from build123d import *

# Parameters (mm, degrees)
SHELL1_T  = -0.1
SKETCH4_W = 5
SKETCH4_H = 6


with BuildPart() as part:
    # Sketch3 → Revolve1 (revolve)
    with BuildSketch(Plane.XY):
        with BuildLine():
            Line((0, 0), (5, 0))
            ThreePointArc((5, 0), (3.535533906, 3.535533906), (0, 5))
            Line((0, 5), (0, 0))
        make_face()
    revolve(axis=Axis((0, 0, 0), (0, 1, 0)))

    # Shell1
    shell1_openings = [part.faces().sort_by_distance(p)[0] for p in [
        (0, 0, 0),
    ]]
    offset(amount=SHELL1_T, openings=shell1_openings, kind=Kind.INTERSECTION)

    # Sketch4 → Revolve2 (revolve)
    with BuildSketch(Plane.XY):
        with Locations((2.5, -3)):
            Rectangle(SKETCH4_W, SKETCH4_H)
    revolve(axis=Axis((0, -6, 0), (0, 1, 0)))


solid = part.part
Design review of the part built by this model. Coordinates are the model's own, in mm. Round coordinates to 2 decimals unless told otherwise and drop trailing zeros. Write each loop counter-clockwise with the first axis right and the second up, starting at its lowest first coordinate (ties: lowest second). Pieces come first, ordered by that corner, then holes. Notation, with made-up numbers: (-33, 8) - (-27, 8) arc R21 ccw to (-27, 33) - close; hole circle Ø11 at (18, -23). An arc over 180 degrees is marked (long way). Use a Markdown table: item, result. Add a question column.
1. Mouldability with a two-part tool opening along Z and no side actions: class faces 1 (the face through (0, 0, 0)), 2 (the face through (0, -6, 0)), 3 (the face through (-1.08, -2.96, 4.88)) as +Z half, -Z half, draft (parallel to the pull), parting line (faces both ways), or undercut.
2. Wall thickness on probe 1 along X at (y, z) = (2.5, -3.5); probe 2 along Y at (x, z) = (-3, -3); probe 3 along X at (y, z) = (0.75, 3.75): over which ranges is each line inside the solid? List them lowest first.
3. We need section A-A (z = 0). State the section outline as (x, y) points, then the cut area to 3 significant figures.
4. We need section B-B (x = -3). State the section outline as (y, z) points.
5. We need section C-C (y = 0.25). State the section outline as (x, z) points.
6. Clearance check with flat-ended pins moving along their axes: pin 1 (2 mm diameter, centred on x = -2, z = 1.5, fed in from +Y); pin 2 (1.5 mm diameter, centred on x = 2, y = 1.5, fed in from +Z). State where each tip first meets the part, or that it passes through.
7. We need section D-D (z = 3). State the section outline as (x, y) points, then the cut area to 3 significant figures.
Output:
| question | item | result |
|---|---|---|
| 1 | face 1 | undercut |
| 1 | face 2 | draft |
| 1 | face 3 | parting line |
| 2 | probe 1 | x = -2.55 to -2.35, 2.35 to 2.55 |
| 2 | probe 2 | y = -6 to 0, 2.45 to 2.65 |
| 2 | probe 3 | x = -3.22 to -3.06, 3.06 to 3.22 |
| 3 | outline | (-5, -6) - (5, -6) - (5, 0) arc R5 ccw to (-5, 0) - close; hole (-4.9, 0) - (4.9, 0) arc R4.9 ccw to start |
| 3 | area | 61.6 mm2 |
| 4 | outline | (-6, -4) - (0, -4) arc R4 ccw to (0, 4) - (-6, 4) - close; hole (0, -3.87) arc R3.87 ccw to (0, 3.87) - close |
| 5 | outline | circle Ø9.99 at (0, 0); hole circle Ø9.79 at (0, 0) |
| 6 | pin 1 | stops at y = 4.77 |
| 6 | pin 2 | stops at z = 4.68 |
| 7 | outline | (-4, -6) - (4, -6) - (4, 0) arc R4 ccw to (-4, 0) - close; hole (-3.87, 0) - (3.87, 0) arc R3.87 ccw to start |
| 7 | area | 49.6 mm2 |
